Source: CAD feature listing. Evaluate the final solid. Frame: model axes, mm. A direction names the side the tool comes from. Give positions to 0.01 mm unless a question says otherwise; leave off trailing zeros. Loops run counter-clockwise (first coordinate to the right, second up) from the corner with the lowest first, then second, coordinate; pieces in that order, holes last.
from build123d import *


with BuildPart() as f1:
    # F0 (on Front) → F1 (revolve)
    with BuildSketch(Plane.XZ):
        Polygon((-74.720278, 14.313716), (-252.520278, 14.313716), (-252.520278, 9.551216), (268.179722, 9.551216), (268.179722, 14.313716), (90.379722, 14.313716), align=None)
        Polygon((-74.720278, 16.536216), (-74.720278, 14.313716), (90.379722, 14.313716), (90.379722, 16.536216), (7.829722, 16.536216), align=None)
    revolve(axis=Axis((7.829722, 0, 9.551216), (1, 0, 0)))


solid = f1.part
1) Cut plane C-C (x = 198). Return loops of the section in (y, z) (1 decimal), and give its area (3 significant figures).
Checks:
outline: circle Ø9.5 at (0, 9.6)
area: 71.3 mm2
2) Cut plane B-B (z = 8.5). Return loops of the section in (x, y).
Checks:
outline: (-252.52, -4.65) - (-74.72, -4.65) - (-74.72, -6.91) - (90.38, -6.91) - (90.38, -4.65) - (268.18, -4.65) - (268.18, 4.65) - (90.38, 4.65) - (90.38, 6.91) - (-74.72, 6.91) - (-74.72, 4.65) - (-252.52, 4.65) - close
3) Cut plane A-A (y = 0). Return loops of the section in (x, z), and give its area (3 significant figures).
Checks:
outline: (-252.52, 4.79) - (-74.72, 4.79) - (-74.72, 2.57) - (90.38, 2.57) - (90.38, 4.79) - (268.18, 4.79) - (268.18, 14.31) - (90.38, 14.31) - (90.38, 16.54) - (-74.72, 16.54) - (-74.72, 14.31) - (-252.52, 14.31) - close
area: 5,690 mm2
4) Ray query, probe 1 along X at (y, z) = (-6, 9.75); probe 2 along Y at (x, z) = (-151, 9.5); probe 3 along Y at (x, z) = (-22.5, 15). Return the intervals inside material, ascending.
Checks:
probe 1: x = -74.72 to 90.38
probe 2: y = -4.76 to 4.76
probe 3: y = -4.37 to 4.37
5) Reachability of faces 1 (the flat face through (-252.52, 0, 9)), 2 (the cylindrical face through (-164.865, 2.898, 5.772)), 3 (the flat face through (90.38, 5, 8)) from +Z, -Z, +X, -X, +Y, -Y: full face, straight path, thin tool, end or side. Return the list, or none.
Checks:
face 1: +Z, -Z, -X, +Y, -Y
face 2: -X
face 3: +X
6) Contact query for flat-ended pins moving along their axis: P1, Ø5, axis at x = 168.5, z = 15, coming from the -Y side; P2, Ø4, axis at x = -135.5, y = -2, coming from the +Z side; P3, Ø6, axis at x = 33, y = 4.5, coming from the -Z side. Output: stop coordinate, or through.
Checks:
P1: stops at y = -3.74
P2: stops at z = 14.31
P3: stops at z = 2.73
7) Cut plane D-D (x = 39.5). Return loops of the section in (y, z) (3 decimals), and give its area (3 significant figures).
Checks:
outline: circle Ø13.97 at (0, 9.551)
area: 153 mm2
